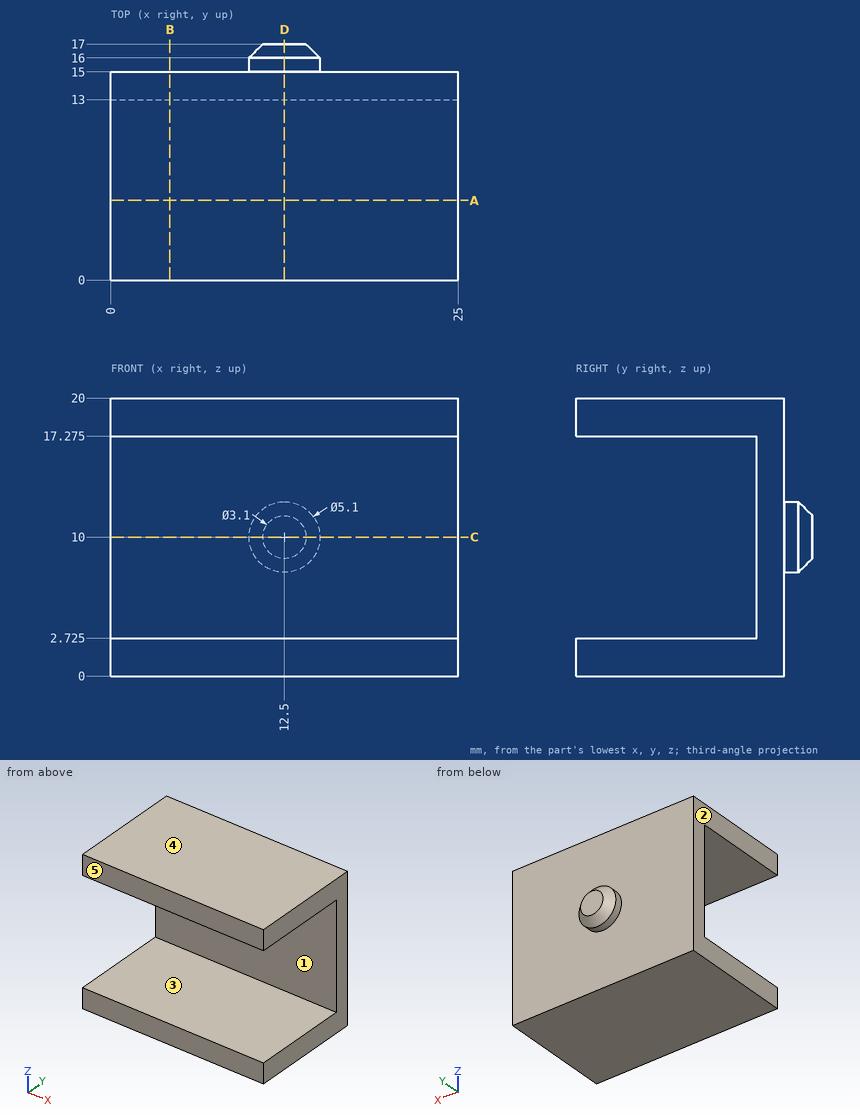
Verification items for this drawing (mm, ordinates from the low corner). A direction names the side the tool comes from. Coordinates: 2 decimals unless noted, no trailing zeros. Write each loop counter-clockwise with the first axis right and the second up, starting at its lowest first coordinate (ties: lowest second). Pieces come first, ordered by that corner, then holes. Notation, with made-up numbers: M -23,17.25 L 3,17.25 A10 cw 3,22.25 Z; hole C -39.5,37.25 d5. An arc over 180 degrees is marked long. Use CSV: the item, a comma, the result in double quotes.
Q1. Section check C-C, the plane z = 10. Enter the section's corners in (x, y).
Computed values:
outline,"M 0,13 L 25,13 L 25,15 L 15.05,15 L 15.05,16 L 14.05,17 L 10.95,17 L 9.95,16 L 9.95,15 L 0,15 Z"
Q2. Set-up check for the marked faces 1 and 2: record each of +Z, -Z, +X, -X, +Y, -Y from which the full face is reachable in a straight line by a thin tool's end or side.
Computed values:
face 1,"+X, -X, -Y"
face 2,"+Z, -Z, -X, +Y, -Y"
Q3. Thickness scan on line 1 along Z through (x, y) = (4, 4.75) (3 decimals); line 2 along Y through (x, z) = (15.25, 16.25); line 3 along Y through (x, z) = (20.75, 19). Record the ranges inside material, lowest first. Write a range as [from, to].
Computed values:
line 1,"[0, 2.725], [17.275, 20]"
line 2,"[13, 15]"
line 3,"[0, 15]"
Q4. Section check A-A, the plane y = 5.75. Enter the section's corners in (x, z) (3 decimals), and give its area (3 significant figures).
Computed values:
outline,"M 0,0 L 25,0 L 25,2.725 L 0,2.725 Z; M 0,17.275 L 25,17.275 L 25,20 L 0,20 Z"
area,"136 mm²"
Q5. Section check D-D, the plane x = 12.5. Enter the section's corners in (y, z) (3 decimals).
Computed values:
outline,"M 0,0 L 15,0 L 15,7.45 L 16,7.45 L 17,8.45 L 17,11.55 L 16,12.55 L 15,12.55 L 15,20 L 0,20 L 0,17.275 L 13,17.275 L 13,2.725 L 0,2.725 Z"
Q6. Go/stop test with flat-tipped pins: P1, Ø1, axis at x = 19.5, z = 9.5, coming from the -Y side; P2, Ø2, axis at x = 17, z = 10, coming from the +Y side. Record where each tip stops, or that it passes through.
Computed values:
P1,"y = 13"
P2,"y = 15"
Q7. Mould release check, pull along Z, two halves, no side actions. Record for the marked faces 3, 4 and 5: pulls with the +Z half, pulls with the -Z half, needs draft (parallel to the pull), parting line crosses it, or undercut.
Computed values:
face 3,"undercut"
face 4,"pulls with the +Z half"
face 5,"needs draft"
Q8. Section check B-B, the plane x = 4.25. Enter the section's corners in (y, z) (3 decimals), and give its area (3 significant figures).
Computed values:
outline,"M 0,0 L 15,0 L 15,20 L 0,20 L 0,17.275 L 13,17.275 L 13,2.725 L 0,2.725 Z"
area,"111 mm²"
